Part model, mm, in its own coordinate system. A direction names the side the tool comes from. Round coordinates to 2 decimals unless told otherwise and drop trailing zeros. Order: outer loops, then holes, each group sorted by start corner. A loop starts at its lowest first (then second) coordinate and runs counter-clockwise, first axis right, second up. Notation, with made-up numbers: (1.5, 40.25) - (38.5, 40.25) arc R27 ccw to (38.5, 70.25) - close; hole circle Ø8 at (-10, 11). An arc over 180 degrees is marked (long way). Return JSON: item names as keys, results as strings. Group by question number.
Item 1: Probe probe 1 along X at (y, z) = (-67.5, 3.5); probe 2 along Y at (x, z) = (-80.5, 4.4); probe 3 along Y at (x, z) = (-67, 1.35). List the from-to ranges inside material, lowest first.
Item 2: Saw through at A-A on y = -76.5. List the corners of the cut face in (x, z), and give its area (3 significant figures).
Item 3: Saw through at C-C on x = -71.5. List the corners of the cut face in (y, z), and give its area (3 significant figures).
Item 4: Saw through at B-B on z = 1.15. List the corners of the cut face in (x, y), and give its area (3 significant figures).
Item 5: Two-plate mould, pull along X, no slides. Class faces 3 (the face through (-81, 7.148, 3)), 4 (the face through (-118.202, -23, 2)), 5 (the face through (-106, -92.852, 2)): released by +X, released by -X, zero draft, split by the parting line, or undercut.
Item 6: Drop flat-ended pins along their axis: pin 1 (5 mm diameter, centred on x = -92.5, y = 3, fed in from -Z); pin 2 (2.5 mm diameter, centred on y = -27, z = 3, fed in from +X); pin 3 (2.5 mm diameter, centred on x = -84, z = 1.5, fed in from -Y); pin 4 (2.5 mm diameter, centred on x = -104.5, z = 2, fed in from -Y). Give the stop position or say it passes through.
Item 7: Tool access for faces 1 (the face through (-68.836, -42, 2)), 2 (the face through (-63, -25, 0)): list every direction of +Z, -Z, +X, -X, +Y, -Y with a clear straight run to the whole face (end or side of a thin tool).
```python
from build123d import *

# Parameters (mm, degrees)
F0_W     = 41.33233428
F0_H     = 35.7883912511
F1_DEPTH = 5
F2_W     = 41.8983511627
F2_H     = 101.1332413182
F3_DEPTH = 5
F4_DEPTH = 25
F5_DEPTH = 25
F6_W     = 25
F6_H     = 100
F7_DEPTH = 5
F8_R     = 5


with BuildPart() as f1:
    # F0 (on Top) → F1 (new body)
    with BuildSketch(Plane.XY):
        with Locations((-47.535456717, 24.881032994)):
            Rectangle(F0_W, F0_H)
    extrude(amount=F1_DEPTH)

    # F2 (on Top) → F3 (join)
    with BuildSketch(Plane.XY):
        with Locations((-47.8867311031, -43.418653775)):
            Rectangle(F2_W, F2_H)
    extrude(amount=F3_DEPTH)

    # F4 (add): a face of the model
    f4_faces = [f1.faces().sort_by_distance(p)[0] for p in [
        (-68.201623857, 24.9615977518, 2.5),
    ]]
    extrude(f4_faces, amount=F4_DEPTH)

    # F5 (add): a face of the model
    f5_faces = [f1.faces().sort_by_distance(p)[0] for p in [
        (-93.201623857, 24.9615977518, 2.5),
    ]]
    extrude(f5_faces, amount=F5_DEPTH)

    # F6 (on Top) → F7 (join)
    with BuildSketch(Plane.XY):
        with Locations((-105.701623857, -42.8520331159)):
            Rectangle(F6_W, F6_H)
    extrude(amount=F7_DEPTH)

    # F8
    f8_edges = [f1.edges().sort_by_distance(p)[0] for p in [
        (-118.201624, -92.852033, 2.5),
        (-93.201624, -92.852033, 2.5),
        (-68.835907, -93.985274, 2.5),
        (-26.937556, -93.985274, 2.5),
    ]]
    fillet(f8_edges, radius=F8_R)


solid = f1.part
```
Filled in:
{
 "1": {"probe 1": "x = -118.2 to -93.2, -68.84 to -26.94", "probe 2": "y = 7.15 to 42.78", "probe 3": "y = -92.86 to 42.78"},
 "2": {"outline": "(-118.2, 0) - (-93.2, 0) - (-93.2, 5) - (-118.2, 5) - close; (-68.84, 0) - (-26.94, 0) - (-26.94, 5) - (-68.84, 5) - close", "area": "334 mm^2"},
 "3": {"outline": "(7.15, 0) - (42.78, 0) - (42.78, 5) - (7.15, 5) - close", "area": "178 mm^2"},
 "4": {"outline": "(-118.2, -87.85) arc R5 ccw to (-113.2, -92.85) - (-98.2, -92.85) arc R5 ccw to (-93.2, -87.85) - (-93.2, 7.15) - (-68.84, 7.15) - (-68.84, -88.99) arc R5 ccw to (-63.84, -93.99) - (-31.94, -93.99) arc R5 ccw to (-26.94, -88.99) - (-26.94, 6.99) - (-26.87, 6.99) - (-26.87, 42.78) - (-118.2, 42.78) - close", "area": "9,970 mm^2"},
 "5": {"face 3": "undercut", "face 4": "released by -X", "face 5": "zero draft"},
 "6": {"pin 1": "stops at z = 0", "pin 2": "stops at x = -26.94", "pin 3": "stops at y = 7.15", "pin 4": "stops at y = -92.85"},
 "7": {"face 1": "+Z, -Z, -Y", "face 2": "-Z, +X, -X, +Y, -Y"}
}
